Could you check a few things on this drawing? It's one solid part, dimensions in mm from its lowest x, y, z. Round coordinates to 2 decimals unless told otherwise and drop trailing zeros. Write each loop counter-clockwise with the first axis right and the second up, starting at its lowest first coordinate (ties: lowest second). Pieces come first, ordered by that corner, then holes. Notation, with made-up numbers: M -32,89.25 L 0,89.25 A20 cw 0,120.25 Z; hole C 38.5,-18.5 d11. An arc over 180 degrees is marked long. One line per item, written item: value. Start each with the question number.
(1) I want a section at B-B on x = 101.5. Please give me the cut outline in (y, z), and give its area (3 significant figures).
(2) I want a section at A-A on z = 144. Please give me the cut outline in (x, y).
(3) If I drill on L1, parallel to X at y = 2, z = 148.5; L2, parallel to Z at x = 82.5, y = 1.85; L3, parallel to X at y = 0.5, z = 12, over which ranges is the centre line in solid material (lowest first)?
(4) I want a section at D-D on z = 14.5. Please give me the cut outline in (x, y), and give its area (3 significant figures).
(5) I want a section at C-C on y = 1.6. Please give me the cut outline in (x, z), and give its area (3 significant figures).
(6) I'm going to push flat-ended pins straight in: pin 1 Ø0.9 at (y, z) = (1.5, 141) entering from -X; pin 2 Ø1.5 at (x, y) = (35, 1) entering from +Z; pin 3 Ø1.5 at (x, y) = (167.5, 1) entering from -Z. Where does each tip first touch, or does it pass through?
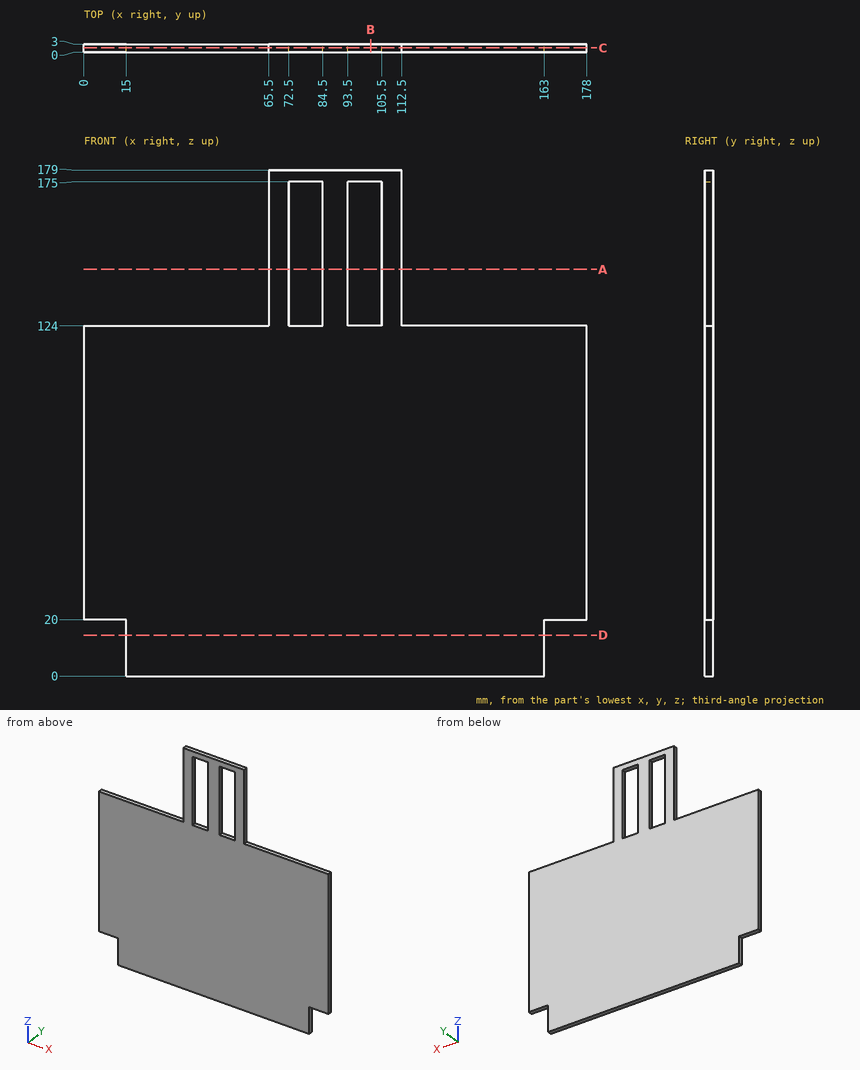
Found:
1. outline: M 0,0 L 3,0 L 3,124 L 0,124 Z; M 0,175 L 3,175 L 3,179 L 0,179 Z
1. area: 384 mm²
2. outline: M 65.5,0 L 72.5,0 L 72.5,3 L 65.5,3 Z; M 84.5,0 L 93.5,0 L 93.5,3 L 84.5,3 Z; M 105.5,0 L 112.5,0 L 112.5,3 L 105.5,3 Z
3. L1: x = 65.5 to 72.5, 84.5 to 93.5, 105.5 to 112.5
3. L2: z = 0 to 124, 175 to 179
3. L3: x = 15 to 163
4. outline: M 15,0 L 163,0 L 163,3 L 15,3 Z
4. area: 444 mm²
5. outline: M 0,20 L 15,20 L 15,0 L 163,0 L 163,20 L 178,20 L 178,124 L 112.5,124 L 112.5,179 L 65.5,179 L 65.5,124 L 0,124 Z; hole M 72.5,124 L 84.5,124 L 84.5,175 L 72.5,175 Z; hole M 93.5,124 L 105.5,124 L 105.5,175 L 93.5,175 Z
5. area: 22,800 mm²
6. pin 1: stops at x = 65.5
6. pin 2: stops at z = 124
6. pin 3: stops at z = 20
